Check sheet for the modelled part. Datum: model origin and axes. Units: mm. Face numbers are marked on the shaded views. Round coordinates to 2 decimals unless told otherwise and drop trailing zeros. Loops run counter-clockwise (first coordinate to the right, second up) from the corner with the lowest first, then second, coordinate; pieces in that order, holes last. Notation, with made-up numbers: (29.25, 19) -> (47.25, 19) arc R18 cw to (47.25, 25) -> close; hole circle Ø11 at (35, 25.25). An arc over 180 degrees is marked (long way). Return JSON: item names as keys, results as strings.
from build123d import *

# Parameters (mm, degrees)
SKETCH1_W           = 101.6
SKETCH1_H           = 19.05
BOSS_EXTRUDE1_DEPTH = 3.175
SKETCH5_R           = 3.175
CUT_EXTRUDE2_DEPTH  = 160.51127542
SKETCH6_W           = 101.6
SKETCH6_H           = 19.05
SKETCH6_R           = 3.175
BOSS_EXTRUDE2_DEPTH = 3.175
SKETCH9_W           = 19.05
SKETCH9_H           = 30.1625
BOSS_EXTRUDE5_DEPTH = 3.175


with BuildPart() as part:
    # Sketch1 → Boss-Extrude1 (new body)
    with BuildSketch(Plane(origin=(0, 0, 0), x_dir=(1, 0, 0), z_dir=(0, 1, 0))):
        with Locations((-104.742582317, 25.692487805)):
            Rectangle(SKETCH1_W, SKETCH1_H)
    extrude(amount=BOSS_EXTRUDE1_DEPTH)

    # Sketch5 → Cut-Extrude2 (cut, through all)
    with BuildSketch(Plane(origin=(0, 3.175, 0), x_dir=(1, 0, 0), z_dir=(0, 1, 0))):
        with Locations(Location((-66.642582317, 25.692487805, 0), (0, 0, 270))):
            Circle(SKETCH5_R)
    extrude(amount=-CUT_EXTRUDE2_DEPTH, mode=Mode.SUBTRACT)



with BuildPart() as body_2:
    # Sketch6 → Boss-Extrude2 (new body)
    with BuildSketch(Plane(origin=(0, 26.9875, 0), x_dir=(1, 0, 0), z_dir=(0, 1, 0))):
        with Locations((-104.742582317, 25.692487805)):
            Rectangle(SKETCH6_W, SKETCH6_H)
        with Locations(Location((-66.642582317, 25.692487805, 0), (0, 0, 270))):
            Circle(SKETCH6_R, mode=Mode.SUBTRACT)
    extrude(amount=BOSS_EXTRUDE2_DEPTH)


with BuildPart() as part_1:
    add(part.part)

    add(body_2.part)  # Boss-Extrude5 merges body 2
    # Sketch9 → Boss-Extrude5 (add)
    with BuildSketch(Plane.ZY.offset(155.542582317)):
        with Locations((-25.692487805, 15.08125)):
            Rectangle(SKETCH9_W, SKETCH9_H)
    extrude(amount=-BOSS_EXTRUDE5_DEPTH)


solid = part_1.part
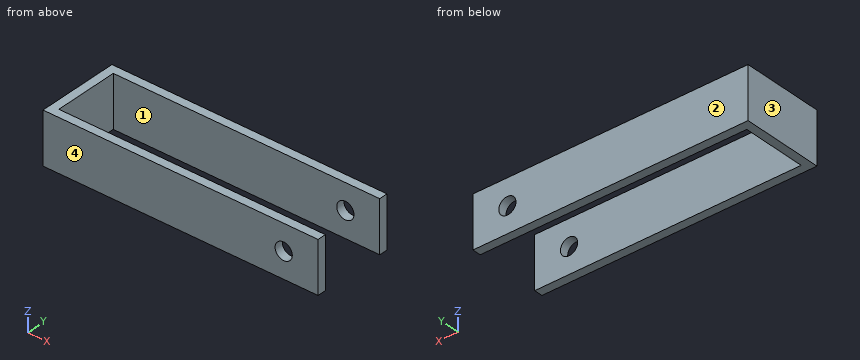
Q1. Material ranges on line 1 (Y direction, x = -101.5, z = -33.5) (1 decimal); line 2 (X direction, y = 18, z = -26); line 3 (X direction, y = 2, z = -28), recorded low to high.
Results list:
{"line 1": "0 to 3.2, 27 to 30.2", "line 2": "-155.54 to -152.37", "line 3": "-155.54 to -68.82, -64.46 to -53.94"}
Q2. Go/stop test with flat-tipped pins: pin 1 (5 mm diameter, centred on x = -117.5, z = -22, fed in from -Y); pin 2 (9.5 mm diameter, centred on y = 15, z = -23, fed in from +X). Record where each tip stops, or that it passes through.
Results list:
{"pin 1": "y = 0", "pin 2": "x = -152.37"}
Q3. Section check D-D (y = 21). Record the boundary of the cut face in (x, z), then the cut area to 3 significant figures.
Results list:
{"outline": "(-155.54, -35.22) -> (-152.37, -35.22) -> (-152.37, -16.17) -> (-155.54, -16.17) -> close", "area": "60.5 mm^2"}
Q4. Section check A-A (x = -124.5). Record the boundary of the cut face in (y, z) (1 decimal), then the cut area to 3 significant figures.
Results list:
{"outline": "(0, -35.2) -> (3.2, -35.2) -> (3.2, -16.2) -> (0, -16.2) -> close; (27, -35.2) -> (30.2, -35.2) -> (30.2, -16.2) -> (27, -16.2) -> close", "area": "121 mm^2"}
Q5. Draft check along Y on the marked faces 1, 2, 3 and 4. Enter one of: released by +Y, released by -Y, zero draft, split by the parting line, or undercut.
Results list:
{"face 1": "undercut", "face 2": "released by +Y", "face 3": "zero draft", "face 4": "released by -Y"}
Q6. Section check C-C (z = -26). Record the boundary of the cut face in (x, y) (1 decimal).
Results list:
{"outline": "(-155.5, 0) -> (-69.8, 0) -> (-69.8, 3.2) -> (-152.4, 3.2) -> (-152.4, 27) -> (-69.8, 27) -> (-69.8, 30.2) -> (-155.5, 30.2) -> close; (-63.5, 0) -> (-53.9, 0) -> (-53.9, 3.2) -> (-63.5, 3.2) -> close; (-63.5, 27) -> (-53.9, 27) -> (-53.9, 30.2) -> (-63.5, 30.2) -> close"}
Q7. Section check B-B (z = -18.75). Record the boundary of the cut face in (x, y) (1 decimal), then the cut area to 3 significant figures.
Results list:
{"outline": "(-155.5, 0) -> (-53.9, 0) -> (-53.9, 3.2) -> (-152.4, 3.2) -> (-152.4, 27) -> (-53.9, 27) -> (-53.9, 30.2) -> (-155.5, 30.2) -> close", "area": "721 mm^2"}
